Source: three-view drawing plus pictorial views. Frame: mm from the lowest corner of the part. A direction names the side the tool comes from. Give positions to 0.01 mm unless a question says otherwise; leave off trailing zeros. Write each loop counter-clockwise with the first axis right and the second up, starting at its lowest first coordinate (ties: lowest second). Pieces come first, ordered by that corner, then holes. Notation, with made-up numbers: M 35.25,46 L 72.25,46 A30 cw 72.25,82 Z; hole C 60,82.25 d5. An arc over 180 degrees is marked long. One line per question, with ' | ' between items.
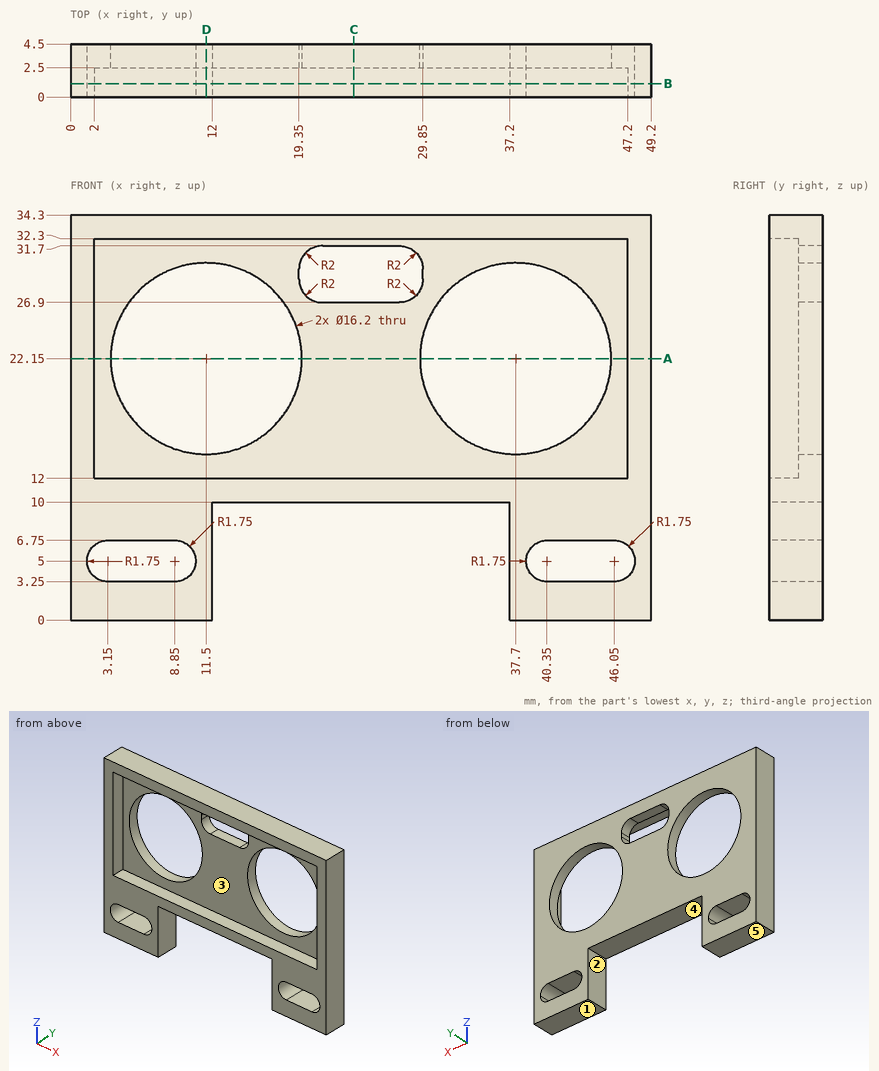
(1) First-contact query: P1, Ø4, axis at x = 41, z = 8, coming from the -Y side. Flat tip, straight axial feed; report the tip coordinate or a pass-through.
Working result:
P1: stops at y = 0
(2) Cut plane A-A, the plane z = 22.15. Return loops of the section in (x, y), then the cut area to 3 significant figures.
Working result:
outline: M 0,0 L 2,0 L 2,2.5 L 3.4,2.5 L 3.4,4.5 L 0,4.5 Z; M 19.6,2.5 L 29.6,2.5 L 29.6,4.5 L 19.6,4.5 Z; M 45.8,2.5 L 47.2,2.5 L 47.2,0 L 49.2,0 L 49.2,4.5 L 45.8,4.5 Z | area: 43.6 mm^2
(3) Material intervals for L1, parallel to Z at x = 25.5, y = 1.35; L2, parallel to Z at x = 28, y = 3; L3, parallel to X at y = 0.6, z = 22.5, sorted ascending. Write a range as [from, to].
Working result:
L1: z = [10, 12], [32.3, 34.3] | L2: z = [10, 26.91], [31.69, 34.3] | L3: x = [0, 2], [47.2, 49.2]
(4) Draft query along Z for the marked faces 1, 2 and 3. Return one class per face: released by +Z, released by -Z, zero draft, split by the parting line, or undercut.
Working result:
face 1: released by -Z | face 2: zero draft | face 3: undercut
(5) Cut plane C-C, the plane x = 24. Return loops of the section in (y, z).
Working result:
outline: M 0,10 L 4.5,10 L 4.5,26.9 L 2.5,26.9 L 2.5,12 L 0,12 Z; M 0,32.3 L 2.5,32.3 L 2.5,31.7 L 4.5,31.7 L 4.5,34.3 L 0,34.3 Z
(6) Set-up query: the marked faces 4 and 5. Return all of +Z, -Z, +X, -X, +Y, -Y with unobstructed straight access to the full face (end or side cutting, diameter ignored); none if empty.
Working result:
face 4: -Z, +Y, -Y | face 5: -Z, +X, -X, +Y, -Y
(7) Cut plane B-B, the plane y = 1.15. Return loops of the section in (x, z), then the cut area to 3 significant figures.
Working result:
outline: M 0,0 L 12,0 L 12,10 L 37.2,10 L 37.2,0 L 49.2,0 L 49.2,34.3 L 0,34.3 Z; hole M 2,12 L 47.2,12 L 47.2,32.3 L 2,32.3 Z; hole M 3.15,3.25 L 8.85,3.25 A1.75 ccw 8.85,6.75 L 3.15,6.75 A1.75 ccw Z; hole M 40.35,3.25 L 46.05,3.25 A1.75 ccw 46.05,6.75 L 40.35,6.75 A1.75 ccw Z | area: 459 mm^2
(8) Cut plane D-D, the plane x = 11.5. Return loops of the section in (y, z).
Working result:
outline: M 0,0 L 4.5,0 L 4.5,14.05 L 2.5,14.05 L 2.5,12 L 0,12 Z; M 0,32.3 L 2.5,32.3 L 2.5,30.25 L 4.5,30.25 L 4.5,34.3 L 0,34.3 Z
